Read the model definition and answer for the solid it produces. Units are mm, in the model's axes. Give positions to 0.01 mm unless a question says otherwise; leave off trailing zeros. Write each loop counter-clockwise with the first axis right and the second up, starting at its lowest first coordinate (ties: lowest second). Pieces come first, ordered by that corner, then holes. Notation, with made-up numbers: (21, -23) -> (46, -23) arc R20 cw to (46, -9) -> close; hole circle Ø10 at (14, -7.5). An arc over 180 degrees is marked (long way). Use a Markdown table: item, result.
from build123d import *

# Parameters (mm, degrees)
SKETCH1_R           = 10
BOSS_EXTRUDE1_DEPTH = 205
SKETCH2_W           = 5
SKETCH2_H           = 23.07
CUT_EXTRUDE1_DEPTH  = 20


with BuildPart() as part:
    # Sketch1 → Boss-Extrude1 (new body)
    with BuildSketch(Plane(origin=(0, 0, 0), x_dir=(1, 0, 0), z_dir=(0, 1, 0))):
        with Locations(Location((0, 0, 0), (0, 0, 90))):
            Circle(SKETCH1_R)
    extrude(amount=BOSS_EXTRUDE1_DEPTH)

    # Sketch2 → Cut-Extrude1 (cut)
    with BuildSketch(Plane(origin=(0, 205, 0), x_dir=(1, 0, 0), z_dir=(0, 1, 0))):
        Rectangle(SKETCH2_W, SKETCH2_H)
    extrude(amount=-CUT_EXTRUDE1_DEPTH, mode=Mode.SUBTRACT)


solid = part.part
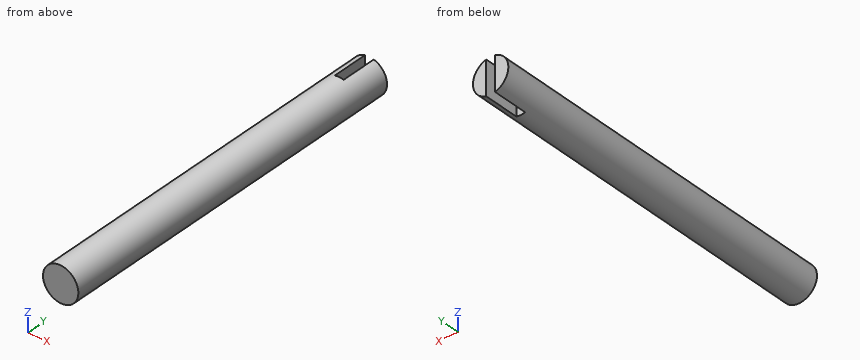
Item 1: Straight lines are drawn through the part: line 1 along Y through (x, z) = (-0.75, -7.5); line 2 along Z through (x, y) = (-2.5, 165.5); line 3 along X through (y, z) = (193.5, -5.5). For each, find the intervals that lie inside material, in ascending order. Write a range as [from, to].
Return value:
| item | result |
|---|---|
| line 1 | [0, 185] |
| line 2 | [-9.68, 9.68] |
| line 3 | [-8.35, -2.5], [2.5, 8.35] |
Item 2: A cutting plane is placed at A-A (z = 0). Give the vertices of the cut face in (x, y), then the cut area to 3 significant figures.
Return value:
| item | result |
|---|---|
| outline | (-10, 0) -> (10, 0) -> (10, 205) -> (2.5, 205) -> (2.5, 185) -> (-2.5, 185) -> (-2.5, 205) -> (-10, 205) -> close |
| area | 4,000 mm^2 |
Item 3: Each of these flat-tipped pins is pushed along its axis until it touches: P1, Ø1, axis at x = -7.5, y = 87, coming from the -Z side; P2, Ø12, axis at y = 27, z = 5.5, coming from the -X side; P3, Ø4, axis at y = 62.5, z = -4.5, coming from the -X side; P4, Ø2, axis at x = -5, y = 157, coming from the -Z side. Where does it stop, or does it pass through?
Return value:
| item | result |
|---|---|
| P1 | z = -7.14 |
| P2 | x = -10 |
| P3 | x = -9.68 |
| P4 | z = -9.17 |
Item 4: A cutting plane is placed at B-B (y = 147.5). Give the vertices of the cut face in (x, z), then the cut area to 3 significant figures.
Return value:
| item | result |
|---|---|
| outline | circle Ø20 at (0, 0) |
| area | 314 mm^2 |
Item 5: A cutting plane is placed at D-D (x = 7.25). Give the vertices of the cut face in (y, z), then the cut area to 3 significant figures.
Return value:
| item | result |
|---|---|
| outline | (0, -6.89) -> (205, -6.89) -> (205, 6.89) -> (0, 6.89) -> close |
| area | 2,820 mm^2 |
Item 6: A cutting plane is placed at C-C (x = 0). Give the vertices of the cut face in (y, z), then the cut area to 3 significant figures.
Return value:
| item | result |
|---|---|
| outline | (0, -10) -> (185, -10) -> (185, 10) -> (0, 10) -> close |
| area | 3,700 mm^2 |
